The model under review builds one solid part; all positions refer to its coordinate system, in mm. Face numbers are marked on the shaded views. A direction names the side the tool comes from. Round coordinates to 2 decimals unless told otherwise and drop trailing zeros. Write each loop counter-clockwise with the first axis right and the second up, starting at its lowest first coordinate (ties: lowest second). Pieces come first, ordered by that corner, then holes. Notation, with made-up numbers: (42, 54) - (46, 54) arc R19 cw to (46, 90) - close; hole circle Ø6 at (-15.5, 58). An arc over 180 degrees is marked (long way). Return JSON: item names as keys, results as strings.
from build123d import *

# Parameters (mm, degrees)
SKETCH2_R          = 14.510934511
CUT_EXTRUDE1_DEPTH = 1.2
SKETCH3_R          = 1.106535356
CUT_EXTRUDE2_DEPTH = 95.2
SKETCH4_R          = 9.062497532
CUT_EXTRUDE3_DEPTH = 1


with BuildPart() as part:
    # Sketch1 → Revolve1 (revolve)
    with BuildSketch(Plane.XY, mode=Mode.PRIVATE) as revolve1_sk:
        with BuildLine():
            Line((0, 0), (0, 84.55))
            Line((0, 84.55), (3.18, 84.55))
            Line((3.18, 84.55), (3.18, 17.954698654))
            ThreePointArc((3.18, 17.954698654), (9.896609701, 5.315721242), (24.13, 3.81))
            Line((24.13, 3.81), (26.67, 1.27))
            Line((26.67, 1.27), (26.67, 0))
            Line((26.67, 0), (0, 0))
        make_face()
    revolve(revolve1_sk.sketch.rotate(Axis((0, 0, 0), (0, 1, 0)), 90), axis=Axis((0, 0, 0), (0, 1, 0)))

    # Sketch2 → Cut-Extrude1 (cut)
    with BuildSketch(Plane.XZ):
        with Locations(Location((0, 0, 0), (0, 0, 270))):
            Circle(SKETCH2_R)
    extrude(amount=-CUT_EXTRUDE1_DEPTH, mode=Mode.SUBTRACT)

    # Sketch3 → Cut-Extrude2 (cut)
    with BuildSketch(Plane(origin=(0, 84.55, 0), x_dir=(1, 0, 0), z_dir=(0, 1, 0))):
        with Locations(Location((0, 0, 0), (0, 0, 270))):
            Circle(SKETCH3_R)
    extrude(amount=-CUT_EXTRUDE2_DEPTH, mode=Mode.SUBTRACT)

    # Sketch4 → Cut-Extrude3 (cut)
    with BuildSketch(Plane.XZ.offset(-1.2)):
        with Locations(Location((0, 0, 0), (0, 0, 270))):
            Circle(SKETCH4_R)
    extrude(amount=-CUT_EXTRUDE3_DEPTH, mode=Mode.SUBTRACT)


solid = part.part
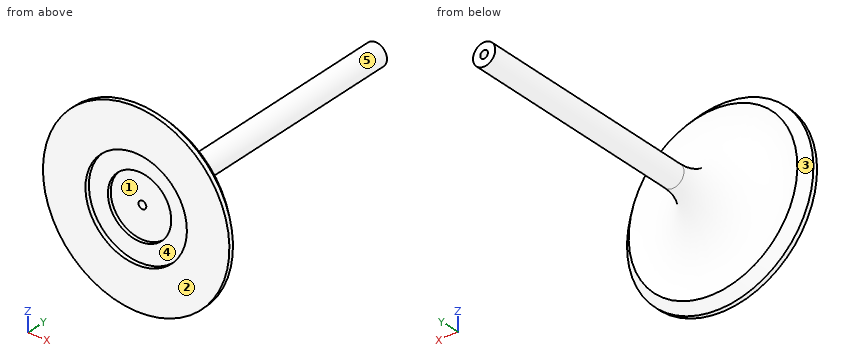
(1) Wall thickness on line 1 (X direction, y = 68, z = 0); line 2 (X direction, y = 1, z = 0); line 3 (Y direction, x = 11.5, z = 9): over which ranges is each line inside the solid? List them lowest first.
Filled in:
{"line 1": "x = -3.18 to -1.11, 1.11 to 3.18", "line 2": "x = -26.67 to -14.51, 14.51 to 26.67", "line 3": "y = 0 to 3.19"}
(2) Add section C-C (y = 50). Write out the cut boundary in (x, z).
Filled in:
{"outline": "circle Ø6.36 at (0, 0); hole circle Ø2.21 at (0, 0)"}
(3) Mouldability with a two-part tool opening along X and no side actions: class the marked faces 1, 2 and 3 as released by +X, released by -X, zero draft, split by the parting line, or undercut.
Filled in:
{"face 1": "undercut", "face 2": "zero draft", "face 3": "split by the parting line"}
(4) Add section A-A (x = 0). Write out the cut boundary in (y, z), plus the area to 3 significant figures.
Filled in:
{"outline": "(0, -26.67) - (1.27, -26.67) - (3.81, -24.13) arc R15.25 cw to (17.95, -3.18) - (84.55, -3.18) - (84.55, -1.11) - (2.2, -1.11) - (2.2, -9.06) - (1.2, -9.06) - (1.2, -14.51) - (0, -14.51) - close; (0, 14.51) - (1.2, 14.51) - (1.2, 9.06) - (2.2, 9.06) - (2.2, 1.11) - (84.55, 1.11) - (84.55, 3.18) - (17.95, 3.18) arc R15.25 cw to (3.81, 24.13) - (1.27, 26.67) - (0, 26.67) - close", "area": "533 mm2"}
(5) Add section D-D (y = 9.5). Write out the cut boundary in (x, z).
Filled in:
{"outline": "circle Ø11.48 at (0, 0); hole circle Ø2.21 at (0, 0)"}
(6) For the marked faces 4 and 5, list the 3-axis set-ups (+Z, -Z, +X, -X, +Y, -Y) from which the entire face can be reached by the end or side of a thin tool; tool diameter is ignored.
Filled in:
{"face 4": "-Y", "face 5": "+Y"}
(7) Clearance check with flat-ended pins moving along their axes: pin 1 Ø20 at (x, z) = (1.5, 1) entering from -Y; pin 2 Ø4 at (x, z) = (-11, -1) entering from +Y; pin 3 Ø1 at (x, z) = (-0.5, -17.5) entering from +Y. State where each tip first meets the part, or that it passes through.
Filled in:
{"pin 1": "stops at y = 1.2", "pin 2": "stops at y = 5.93", "pin 3": "stops at y = 2.77"}
(8) Add section B-B (z = 0). Write out the cut boundary in (x, y).
Filled in:
{"outline": "(-26.67, 0) - (-14.51, 0) - (-14.51, 1.2) - (-9.06, 1.2) - (-9.06, 2.2) - (-1.11, 2.2) - (-1.11, 84.55) - (-3.18, 84.55) - (-3.18, 17.95) arc R15.25 cw to (-24.13, 3.81) - (-26.67, 1.27) - close; (1.11, 2.2) - (9.06, 2.2) - (9.06, 1.2) - (14.51, 1.2) - (14.51, 0) - (26.67, 0) - (26.67, 1.27) - (24.13, 3.81) arc R15.25 cw to (3.18, 17.95) - (3.18, 84.55) - (1.11, 84.55) - close"}
